Model file for the job. Use its own axes, mm. Give positions to 0.01 mm unless a question says otherwise; leave off trailing zeros. Loops run counter-clockwise (first coordinate to the right, second up) from the corner with the lowest first, then second, coordinate; pieces in that order, holes last. Notation, with made-up numbers: M 89,33.25 L 100,33.25 A20 cw 100,43.25 Z; hole C 60,67 d10. An arc over 180 degrees is marked long. Answer in a Markdown table with one row per item.
```python
from build123d import *

# Parameters (mm, degrees)
SKETCH1_W           = 79.31
SKETCH1_H           = 3.17
BOSS_EXTRUDE1_DEPTH = 198
SKETCH2_W           = 3.17
SKETCH2_H           = 118.22
BOSS_EXTRUDE2_DEPTH = 63.76
SKETCH3_W           = 3.17
SKETCH3_H           = 198
BOSS_EXTRUDE3_DEPTH = 48
CUT_EXTRUDE1_DEPTH  = 200


with BuildPart() as part:
    # Sketch1 → Boss-Extrude1 (new body)
    with BuildSketch(Plane(origin=(0, 0, 0), x_dir=(1, 0, 0), z_dir=(0, 1, 0))):
        with Locations((39.655, 1.585)):
            Rectangle(SKETCH1_W, SKETCH1_H)
    extrude(amount=BOSS_EXTRUDE1_DEPTH)

    # Sketch2 → Boss-Extrude2 (add)
    with BuildSketch(Plane.ZY):
        with Locations((-1.585, 99)):
            Rectangle(SKETCH2_W, SKETCH2_H)
    extrude(amount=BOSS_EXTRUDE2_DEPTH)

    # Sketch3 → Boss-Extrude3 (add)
    with BuildSketch(Plane(origin=(79.31, 0, 0), x_dir=(0, 0, -1), z_dir=(1, 0, 0))):
        with Locations((1.585, 99)):
            Rectangle(SKETCH3_W, SKETCH3_H)
    extrude(amount=BOSS_EXTRUDE3_DEPTH)

    # Sketch5 → Cut-Extrude1 (cut)
    with BuildSketch(Plane(origin=(0, 198, 0), x_dir=(1, 0, 0), z_dir=(0, 1, 0))):
        Polygon((124.301364544, 0), (127.332496868, 0.810264437), (127.332496868, 0), align=None)
    extrude(amount=-CUT_EXTRUDE1_DEPTH, mode=Mode.SUBTRACT)


solid = part.part
```
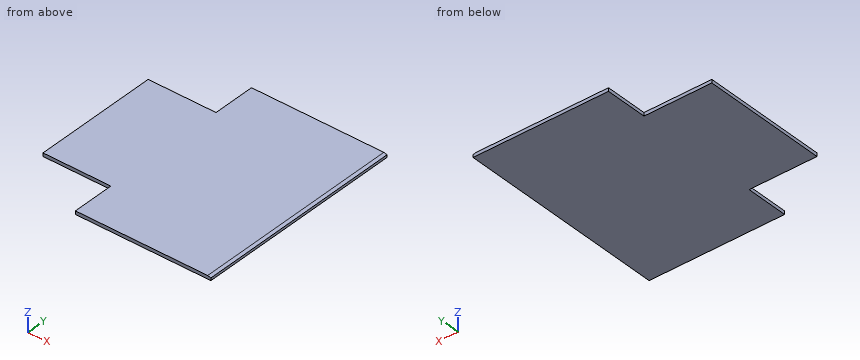
(1) Wall check: L1, parallel to X at y = 166, z = -1.3; L2, parallel to Y at x = -52.5, z = -2.1. Give the ranges that are in metal, low to high.
Established:
| item | result |
|---|---|
| L1 | x = 0 to 127.31 |
| L2 | y = 39.89 to 158.11 |
(2) Saw through at B-B, the plane z = -1.8. Give the cut face in (x, y).
Established:
| item | result |
|---|---|
| outline | M -63.76,39.89 L 0,39.89 L 0,0 L 127.31,0 L 127.31,198 L 0,198 L 0,158.11 L -63.76,158.11 Z |
(3) Saw through at C-C, the plane x = -35. Give the cut face in (y, z), and give its area (3 significant figures).
Established:
| item | result |
|---|---|
| outline | M 39.89,-3.17 L 158.11,-3.17 L 158.11,0 L 39.89,0 Z |
| area | 375 mm2 |
(4) Saw through at A-A, the plane y = 36.5. Give the cut face in (x, z), and give its area (3 significant figures).
Established:
| item | result |
|---|---|
| outline | M 0,-3.17 L 127.31,-3.17 L 127.31,-0.8 L 124.3,0 L 0,0 Z |
| area | 402 mm2 |
(5) Flat gauge pins, fed straight in: P1, Ø1.6, axis at x = -28, z = -1, coming from the -Y side; P2, Ø1, axis at y = 26, z = -2, coming from the -X side. Where does each tip first touch, or does it go through?
Established:
| item | result |
|---|---|
| P1 | stops at y = 39.89 |
| P2 | stops at x = 0 |
